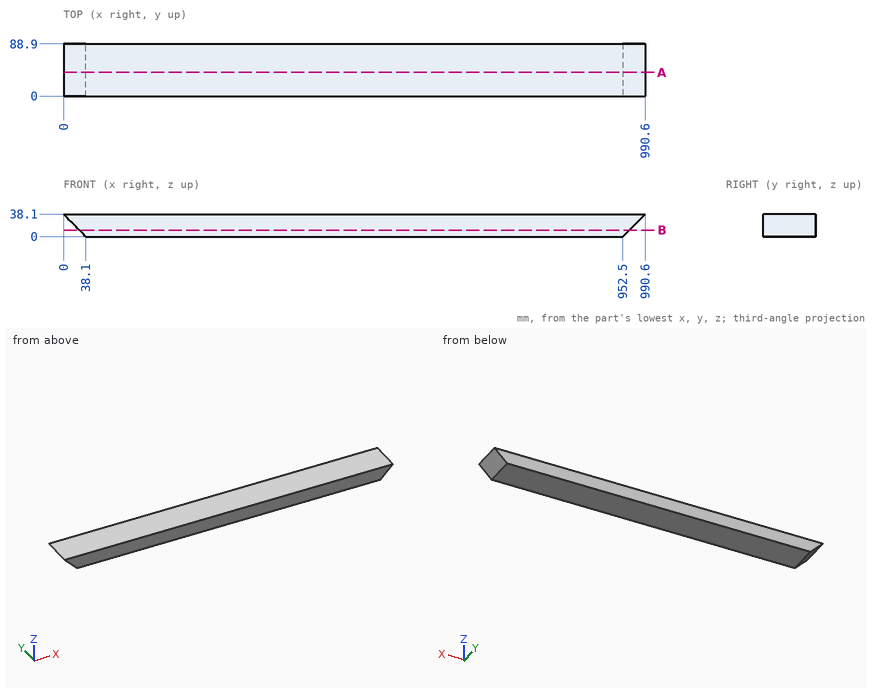
Job drawing, mm, ordinate dimensions from the low corner. One solid piece. Round coordinates to 2 decimals unless told otherwise and drop trailing zeros. Loops run counter-clockwise (first coordinate to the right, second up) from the corner with the lowest first, then second, coordinate; pieces in that order, holes last. Notation, with made-up numbers: (18.25, -16.75) -> (45.25, -16.75) arc R22 ccw to (45.25, 9.25) -> close; hole circle Ø3 at (63.5, -3). An arc over 180 degrees is marked (long way). Use a Markdown table: item, result.
1) Cut at B-B, the plane z = 11. List the corners of the cut face in (x, y).
The answers:
| item | result |
|---|---|
| outline | (27.1, 0) -> (963.5, 0) -> (963.5, 88.9) -> (27.1, 88.9) -> close |
2) Cut at A-A, the plane y = 40.5. List the corners of the cut face in (x, z), and give its area (3 significant figures).
The answers:
| item | result |
|---|---|
| outline | (0, 38.1) -> (38.1, 0) -> (952.5, 0) -> (990.6, 38.1) -> close |
| area | 36,300 mm2 |
3) Drop flat-ended pins along their axis: pin 1 Ø4 at (y, z) = (23, 9) entering from -X; pin 2 Ø12 at (y, z) = (53.5, 25.5) entering from -X; pin 3 Ø4 at (y, z) = (63, 32.5) entering from -X. Give the stop position or say it passes through.
The answers:
| item | result |
|---|---|
| pin 1 | stops at x = 27.1 |
| pin 2 | stops at x = 6.6 |
| pin 3 | stops at x = 3.6 |
4) Probe line 1 (X direction, y = 8, z = 26.5); line 2 (X direction, y = 73, z = 12.5). List the from-to ranges inside material, lowest first. Write a range as [from, to].
The answers:
| item | result |
|---|---|
| line 1 | x = [11.6, 979] |
| line 2 | x = [25.6, 965] |
